Can you work these out from the model? Positions are in its coordinate system, mm. A direction names the side the tool comes from. Coordinates: 2 decimals unless noted, no trailing zeros. Order: outer loops, then holes, each group sorted by start corner. A loop starts at its lowest first (then second) coordinate and runs counter-clockwise, first axis right, second up. Notation, with made-up numbers: (10.5, 44) -> (54.5, 44) arc R8 cw to (54.5, 59) -> close; hole circle Ø1 at (-12.5, 67.5). An arc over 180 degrees is marked (long way). Write item = value, one per line.
```python
from build123d import *

# Parameters (mm, degrees)
SKETCH_1_R          = 25
EXTRUDE_1_DEPTH     = 16
SKETCH_2_R          = 5.5
CUT_EXTRUDE_1_DEPTH = 72.324960568
SKETCH_3_R          = 37.5
EXTRUDE_2_DEPTH     = 115
SKETCH_4_R          = 25
CUT_EXTRUDE_2_DEPTH = 135.373546504


with BuildPart() as part:
    # 草图1 → 凸台-拉伸1 (new body)
    with BuildSketch(Plane.XY):
        with BuildLine():
            Line((-34.910600109, 42.5), (34.910600109, 42.5))
            ThreePointArc((34.910600109, 42.5), (55, 0), (34.910600109, -42.5))
            Line((34.910600109, -42.5), (-34.910600109, -42.5))
            ThreePointArc((-34.910600109, -42.5), (-55, 0), (-34.910600109, 42.5))
        make_face()
        Circle(SKETCH_1_R, mode=Mode.SUBTRACT)
    extrude(amount=EXTRUDE_1_DEPTH)

    # 草图2 → 切除-拉伸1 (cut, through all)
    with BuildSketch(Plane.XY.offset(16)):
        with Locations((-31.723911196, 32.908104345)):
            Circle(SKETCH_2_R)
        with Locations((-43.927765176, 12.637298755)):
            Circle(SKETCH_2_R)
        with Locations((-44.361209952, -11.019660831)):
            Circle(SKETCH_2_R)
        with Locations((-32.908104345, -31.723911196)):
            Circle(SKETCH_2_R)
        with Locations(Location((32.908104345, -31.723911196, 0), (0, 0, 180))):
            Circle(SKETCH_2_R)
        with Locations(Location((44.361209952, -11.019660831, 0), (0, 0, 180))):
            Circle(SKETCH_2_R)
        with Locations(Location((43.927765176, 12.637298755, 0), (0, 0, 180))):
            Circle(SKETCH_2_R)
        with Locations(Location((31.723911196, 32.908104345, 0), (0, 0, 180))):
            Circle(SKETCH_2_R)
    extrude(amount=-CUT_EXTRUDE_1_DEPTH, mode=Mode.SUBTRACT)

    # 草图3 → 凸台-拉伸2 (add)
    with BuildSketch(Plane(origin=(0, 0, 0), x_dir=(-1, 0, 0), z_dir=(0, 0, -1))):
        with Locations(Location((0, 0, 0), (0, 0, 180))):
            Circle(SKETCH_3_R)
    extrude(amount=EXTRUDE_2_DEPTH)

    # 草图4 → 切除-拉伸2 (cut, through all)
    with BuildSketch(Plane.XY):
        Circle(SKETCH_4_R)
    extrude(amount=-CUT_EXTRUDE_2_DEPTH, mode=Mode.SUBTRACT)


solid = part.part
```
Item 1: I want a section at B-B, the plane y = 0. Please give me the cut outline in (x, z).
A:
outline = (-55, 0) -> (-37.5, 0) -> (-37.5, -115) -> (-25, -115) -> (-25, 16) -> (-55, 16) -> close; (25, -115) -> (37.5, -115) -> (37.5, 0) -> (55, 0) -> (55, 16) -> (25, 16) -> close
Item 2: For faces 1 (the cylindrical face through (17.3, 33.27, -56.7)), 2 (the flat face through (0, 42.5, 8)), which set-ups out of +Z, -Z, +X, -X, +Y, -Y let a thin tool reach every point of the face, with its end or its side?
A:
face_1 = -Z
face_2 = +Z, -Z, +X, -X, +Y
Item 3: I'm going to push flat-ended pins straight in: P1, Ø1, axis at x = -13.5, z = -73.5, coming from the -Y side; P2, Ø2, axis at y = -13, z = -7, coming from the +X side; P3, Ø6.5, axis at x = 32.91, y = -31.72, coming from the +Z side; P4, Ø12.5, axis at x = 44.36, y = -11.02, coming from the -Z side. Where does each tip first touch, or does it pass through?
A:
P1 = -35.17
P2 = 35.53
P3 = through
P4 = 0
Item 4: I want a section at A-A, the plane x = 0. Please give me the cut outline in (y, z).
A:
outline = (-42.5, 0) -> (-37.5, 0) -> (-37.5, -115) -> (-25, -115) -> (-25, 16) -> (-42.5, 16) -> close; (25, -115) -> (37.5, -115) -> (37.5, 0) -> (42.5, 0) -> (42.5, 16) -> (25, 16) -> close
Item 5: If we mould it in two halves opening along X, with no side actions, what happens to faces 3 (the cylindrical face through (-33.62, -26.27, 8.11)), 4 (the flat face through (8, 24, -115)), 5 (the cylindrical face through (54.996, 0.68, 7.888))? For each: pulls with the +X half, pulls with the -X half, needs draft (parallel to the pull), parting line crosses it, or undercut.
A:
face_3 = undercut
face_4 = needs draft
face_5 = pulls with the +X half
Item 6: I want a section at C-C, the plane x = 44. Please give me the cut outline in (y, z), plus the area to 3 significant figures.
A:
outline = (-33, 0) -> (-16.51, 0) -> (-16.51, 16) -> (-33, 16) -> close; (-5.53, 0) -> (7.14, 0) -> (7.14, 16) -> (-5.53, 16) -> close; (18.14, 0) -> (33, 0) -> (33, 16) -> (18.14, 16) -> close
area = 704 mm2
Item 7: If I drill on probe 1 along Y at (x, z) = (0, -49); probe 2 along X at (y, z) = (11.5, 3.5); probe 3 along X at (y, z) = (19, -53), over which ranges is the centre line in solid material (lowest first)?
A:
probe_1 = -37.5 to -25, 25 to 37.5
probe_2 = -53.78 to -49.31, -38.55 to -22.2, 22.2 to 38.55, 49.31 to 53.78
probe_3 = -32.33 to -16.25, 16.25 to 32.33
Item 8: I want a section at D-D, the plane z = -27. Please give me the cut outline in (x, y), plus the area to 3 significant figures.
A:
outline = circle Ø75 at (0, 0); hole circle Ø50 at (0, 0)
area = 2,450 mm2
